Input: part model. Units: mm. Frame: model coordinates. A direction names the side the tool comes from. Give positions to 0.01 mm unless a question says otherwise; leave off trailing zeros. Loops run counter-clockwise (first coordinate to the right, second up) from the corner with the lowest first, then second, coordinate; pieces in that order, holes last.
from build123d import *

# Parameters (mm, degrees)
F1_DEPTH = 63.5
F2_DEPTH = 25.4
F3_DEPTH = 7.9375
F5_R     = 12.7


with BuildPart() as f1:
    # F0 (on Front) → F1 (new body, symmetric)
    with BuildSketch(Plane.XZ):
        Polygon((-41.275, 9.525), (-41.275, -9.525), (41.275, -9.525), (41.275, 9.525), (22.225, 9.525), align=None)
    extrude(amount=F1_DEPTH, both=True)

    # F0 (on Front) → F2 (join, symmetric)
    with BuildSketch(Plane.XZ):
        Polygon((85.725, 61.9252), (60.325, 61.9252), (60.325, 42.8752), (85.725, 42.8752), (85.725, 52.3875), align=None)
        with BuildLine():
            Line((22.225, 9.525), (41.275, 9.525))
            Line((41.275, 9.525), (41.275, 27.0002))
            ThreePointArc((41.275, 27.0002), (45.9246798487, 38.2255201513), (57.15, 42.8752))
            Line((57.15, 42.8752), (60.325, 42.8752))
            Line((60.325, 42.8752), (60.325, 61.9252))
            Line((60.325, 61.9252), (57.15, 61.9252))
            add(Edge.make_bspline(
                [(54.8603183175, 61.8500634544), (55.6368577233, 61.8882476927), (56.4004054697, 61.9134098157), (57.15, 61.9252)],
                knots=[109.0783703801, 109.0783703801, 109.0783703801, 109.0783703801, 111.5045361635, 111.5045361635, 111.5045361635, 111.5045361635], degree=3))
            ThreePointArc((54.8603183175, 61.8500634544), (31.6576211608, 50.8726578986), (22.225, 27.0002))
            Line((22.225, 27.0002), (22.225, 9.525))
        make_face()
    extrude(amount=F2_DEPTH, both=True)

    # F0 (on Front) → F3 (join, symmetric)
    with BuildSketch(Plane.XZ):
        with BuildLine():
            add(Edge.make_bspline(
                [(-41.275, 9.525), (-41.2251744093, 32.0946626857), (19.9477606111, 60.1333322619), (54.8603183175, 61.8500634544)],
                knots=[0, 0, 0, 0, 109.0783703801, 109.0783703801, 109.0783703801, 109.0783703801], degree=3))
            Line((-41.275, 9.525), (22.225, 9.525))
            Line((22.225, 9.525), (22.225, 27.0002))
            ThreePointArc((22.225, 27.0002), (31.6576211608, 50.8726578986), (54.8603183175, 61.8500634544))
        make_face()
    extrude(amount=F3_DEPTH, both=True)

    # F0 (on Front) → F4 (revolve)
    with BuildSketch(Plane.XZ):
        Polygon((85.725, 66.675), (85.725, 61.9252), (85.725, 52.3875), (85.725, 42.8752), (85.725, 38.1), (111.125, 38.1), (111.125, 66.675), align=None)
    revolve(axis=Axis((85.725, 0, 45.24375), (0, 0, 1)))

    # F5
    f5_edges = [f1.edges().sort_by_distance(p)[0] for p in [
        (41.275, -63.5, 0),
        (-41.275, -63.5, 0),
        (41.275, 63.5, 0),
        (-41.275, 63.5, 0),
    ]]
    fillet(f5_edges, radius=F5_R)


solid = f1.part
(1) Cut plane A-A (x = 83.5). Return the cut outline in (y, z) (3 decimals), and give its area (3 significant figures).
Values follow:
outline: (-25.4, 42.875) - (-25.302, 42.875) - (-25.302, 38.1) - (25.302, 38.1) - (25.302, 42.875) - (25.4, 42.875) - (25.4, 61.925) - (25.302, 61.925) - (25.302, 66.675) - (-25.302, 66.675) - (-25.302, 61.925) - (-25.4, 61.925) - close
area: 1,450 mm2
(2) Ray query, probe 1 along Y at (x, z) = (33, 53); probe 2 along Z at (x, y) = (30.5, 52.5) (3 decimals); probe 3 along Z at (x, y) = (87, 12.5) (3 decimals). Return the intervals inside material, ascending.
Values follow:
probe 1: y = -7.94 to 7.94
probe 2: z = -9.525 to 9.525
probe 3: z = 38.1 to 66.675
(3) Mould query, pull axis X, two halves, no side actions, for faces 1 (the cylindrical face through (37.653, 59.681, 0.133)), 2 (the flat face through (60, 2, 42.875)), 3 (the flat face through (22.225, 17, 18)), 4 (the flat face through (46, 25.4, 42)). Classes: +X half, -X half, draft (parallel to the pull), parting line (faces both ways), or undercut.
Values follow:
face 1: +X half
face 2: undercut
face 3: -X half
face 4: draft
(4) Pin query (flat end, axial travel): pin 1 Ø5 at (y, z) = (-18, 18.5) entering from -X (3 decimals); pin 2 Ø15.5 at (x, z) = (30, 43) entering from -Y; pin 3 Ø16.5 at (x, y) = (1.5, 24) entering from +Z (3 decimals); pin 4 Ø2 at (y, z) = (27, 50) entering from -X. Return the tip coordinate at first contact, or that it passes through.
Values follow:
pin 1: stops at x = 22.225
pin 2: stops at y = -25.4
pin 3: stops at z = 9.525
pin 4: passes through
(5) Cut plane C-C (x = 102). Return the cut outline in (y, z) (3 decimals).
Values follow:
outline: (-19.501, 38.1) - (19.501, 38.1) - (19.501, 66.675) - (-19.501, 66.675) - close
(6) Cut plane B-B (y = -53). Return the cut outline in (x, z) (3 decimals), and give its area (3 significant figures).
Values follow:
outline: (-41.083, -9.525) - (41.083, -9.525) - (41.083, 9.525) - (-41.083, 9.525) - close
area: 1,570 mm2
(7) Reachability of faces 5 (the flat face through (46, -25.4, 42)), 6 (the flat face through (41.275, -1, 4)), 7 (the flat face through (22.225, -17, 18)), 8 (the flat face through (-3, 7.938, 30)) from +Z, -Z, +X, -X, +Y, -Y: full face, straight path, thin tool, end or side. Return the list, or none.
Values follow:
face 5: +Z, +X, -X, -Y
face 6: -Z, +X, +Y, -Y
face 7: +Z, -X, -Y
face 8: +Z, -X, +Y
